Check sheet for the drawn part. Datum: minimum x, y, z corner. Units: mm. A direction names the side the tool comes from. Coordinates: 2 decimals unless noted, no trailing zeros. Order: outer loops, then holes, each group sorted by start corner. A loop starts at its lowest first (then second) coordinate and runs counter-clockwise, first axis right, second up. Notation, with made-up numbers: M 29.5,48.5 L 83.5,48.5 A13 ccw 83.5,60.5 Z; hole C 59.25,47.5 d5. An arc over 180 degrees is marked long. Return JSON: item names as keys, results as strings. Group by question number.
Q1. Thickness scan on probe 1 along Y at (x, z) = (16, 41); probe 2 along Z at (x, y) = (11, 9.5). Record the ranges inside material, lowest first.
Q2. Section check A-A, the plane x = 16. Enter the section's corners in (y, z), then the cut area to 3 significant figures.
Q3. Go/stop test with flat-tipped pins: pin 1 Ø6 at (y, z) = (10.5, 17.5) entering from +X; pin 2 Ø8 at (y, z) = (16.5, 40) entering from -X; pin 3 Ø6 at (x, y) = (23.5, 9.5) entering from +Z; pin 4 Ø13 at (x, z) = (16, 37) entering from +Y. Record where each tip stops, or that it passes through.
Q4. Section check C-C, the plane y = 4. Enter the section's corners in (x, z), then the cut area to 3 significant figures.
Q5. Access from +Z, -Z, +X, -X, +Y, -Y to the whole of each face (thin tool, end or side, straight path). Record for the marked faces 1, 2 and 3.
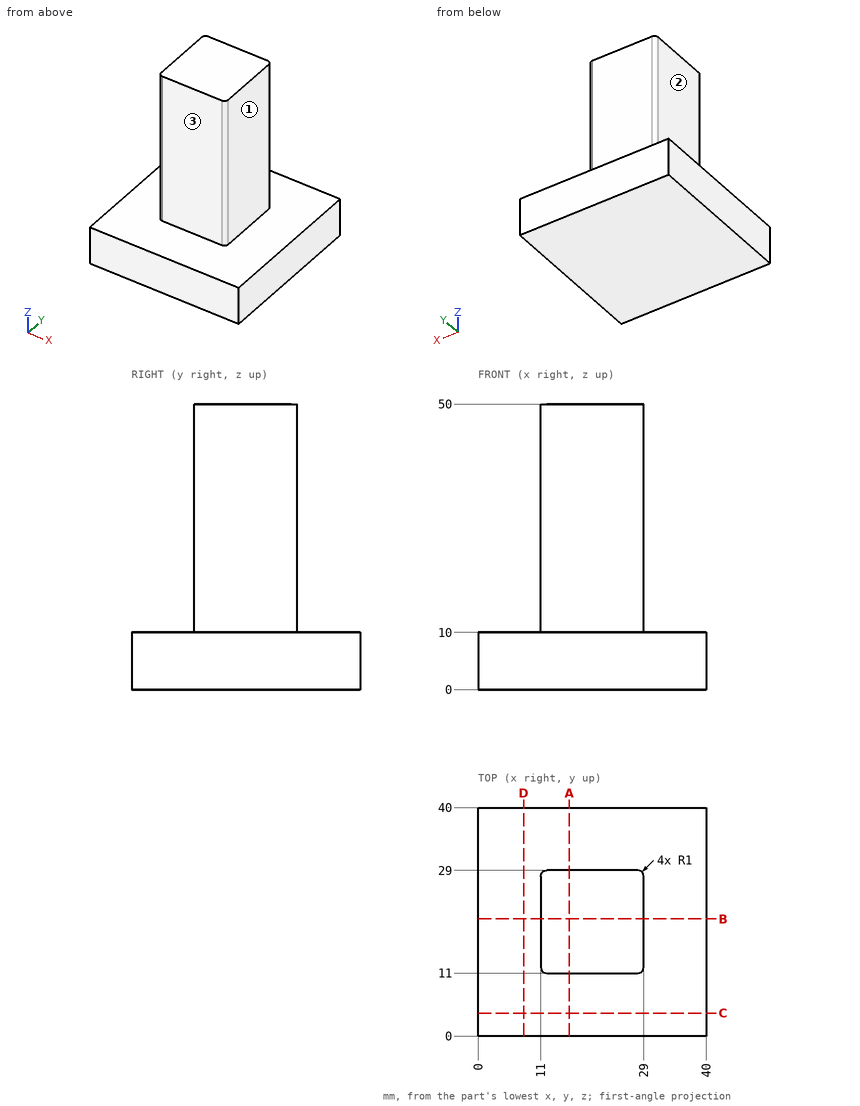
Numbers:
{
 "1": {"probe 1": "y = 11 to 29", "probe 2": "z = 0 to 10"},
 "2": {"outline": "M 0,0 L 40,0 L 40,10 L 29,10 L 29,50 L 11,50 L 11,10 L 0,10 Z", "area": "1,120 mm2"},
 "3": {"pin 1": "stops at x = 29", "pin 2": "stops at x = 11", "pin 3": "stops at z = 50", "pin 4": "stops at y = 29"},
 "4": {"outline": "M 0,0 L 40,0 L 40,10 L 0,10 Z", "area": "400 mm2"},
 "5": {"face 1": "+Z, +X, +Y, -Y", "face 2": "+Z, -X, +Y, -Y", "face 3": "+Z, +X, -X, -Y"}
}
